```python
from build123d import *

# Parameters (mm, degrees)
SKETCH1_W                       = 101.6
SKETCH1_H                       = 114.3
BOSS_EXTRUDE1_DEPTH             = 19.05
SKETCH2_R                       = 30.999938
CUT_EXTRUDE1_DEPTH              = 7.62
SKETCH4_R                       = 15.875
CUT_EXTRUDE2_DEPTH              = 155.110195964
SKETCH5_R                       = 4.0005
CUT_EXTRUDE4_DEPTH              = 155.110195964
SKETCH10_R                      = 7.12499972
CUT_EXTRUDE5_DEPTH              = 7.62
TAP_DRILL_FOR_M8X1_0_TAP2_D     = 7
TAP_DRILL_FOR_M8X1_0_TAP2_DEPTH = 25.4
TAP_DRILL_FOR_M8X1_0_TAP2_TIP   = 2.103012167
TAP_DRILL_FOR_M8X1_0_TAP3_D     = 7
TAP_DRILL_FOR_M8X1_0_TAP3_DEPTH = 25.4
TAP_DRILL_FOR_M8X1_0_TAP3_TIP   = 2.103012167


with BuildPart() as part:
    # Sketch1 → Boss-Extrude1 (new body)
    with BuildSketch(Plane.YZ):
        with Locations((50.8, 57.15)):
            Rectangle(SKETCH1_W, SKETCH1_H)
    extrude(amount=BOSS_EXTRUDE1_DEPTH)

    # Sketch2 → Cut-Extrude1 (cut)
    with BuildSketch(Plane.YZ.offset(19.05)):
        with Locations(Location((50.8, 57.15, 0), (0, 0, 270))):
            Circle(SKETCH2_R)
    extrude(amount=-CUT_EXTRUDE1_DEPTH, mode=Mode.SUBTRACT)

    # Sketch4 → Cut-Extrude2 (cut, through all)
    with BuildSketch(Plane(origin=(0, 0, 0), x_dir=(0, -1, 0), z_dir=(-1, 0, 0))):
        with Locations(Location((-50.8, 57.15, 0), (0, 0, 90))):
            Circle(SKETCH4_R)
    extrude(amount=-CUT_EXTRUDE2_DEPTH, mode=Mode.SUBTRACT)

    # Sketch5 → Cut-Extrude4 (cut, through all)
    with BuildSketch(Plane.YZ.offset(19.05)):
        with Locations(Location((8.382, 99.568, 0), (0, 0, 270))):
            Circle(SKETCH5_R)
        with Locations(Location((93.218, 99.568, 0), (0, 0, 270))):
            Circle(SKETCH5_R)
        with Locations(Location((93.218, 14.732, 0), (0, 0, 270))):
            Circle(SKETCH5_R)
        with Locations(Location((8.382, 14.732, 0), (0, 0, 270))):
            Circle(SKETCH5_R)
    extrude(amount=-CUT_EXTRUDE4_DEPTH, mode=Mode.SUBTRACT)

    # Sketch10 → Cut-Extrude5 (cut)
    with BuildSketch(Plane.YZ.offset(19.05)):
        with Locations(Location((8.382, 99.568, 0), (0, 0, 270))):
            Circle(SKETCH10_R)
        with Locations(Location((93.218, 99.568, 0), (0, 0, 270))):
            Circle(SKETCH10_R)
        with Locations(Location((93.218, 14.732, 0), (0, 0, 270))):
            Circle(SKETCH10_R)
        with Locations(Location((8.382, 14.732, 0), (0, 0, 270))):
            Circle(SKETCH10_R)
    extrude(amount=-CUT_EXTRUDE5_DEPTH, mode=Mode.SUBTRACT)

    # Tap Drill for M8x1.0 Tap2
    with Locations(Plane.XY.offset(114.3)):
        with Locations((9.398, 73.152), (9.398, 28.448)):
            Hole(TAP_DRILL_FOR_M8X1_0_TAP2_D / 2, depth=TAP_DRILL_FOR_M8X1_0_TAP2_DEPTH)
            with Locations((0, 0, -(TAP_DRILL_FOR_M8X1_0_TAP2_DEPTH + TAP_DRILL_FOR_M8X1_0_TAP2_TIP / 2))):  # 118° drill point
                Cone(0, TAP_DRILL_FOR_M8X1_0_TAP2_D / 2, TAP_DRILL_FOR_M8X1_0_TAP2_TIP, mode=Mode.SUBTRACT)

    # Tap Drill for M8x1.0 Tap3
    with Locations(Plane(origin=(0, 0, 0), x_dir=(1, 0, 0), z_dir=(0, 0, -1))):
        with Locations((9.398, -73.152), (9.398, -28.448)):
            Hole(TAP_DRILL_FOR_M8X1_0_TAP3_D / 2, depth=TAP_DRILL_FOR_M8X1_0_TAP3_DEPTH)
            with Locations((0, 0, -(TAP_DRILL_FOR_M8X1_0_TAP3_DEPTH + TAP_DRILL_FOR_M8X1_0_TAP3_TIP / 2))):  # 118° drill point
                Cone(0, TAP_DRILL_FOR_M8X1_0_TAP3_D / 2, TAP_DRILL_FOR_M8X1_0_TAP3_TIP, mode=Mode.SUBTRACT)


solid = part.part
```
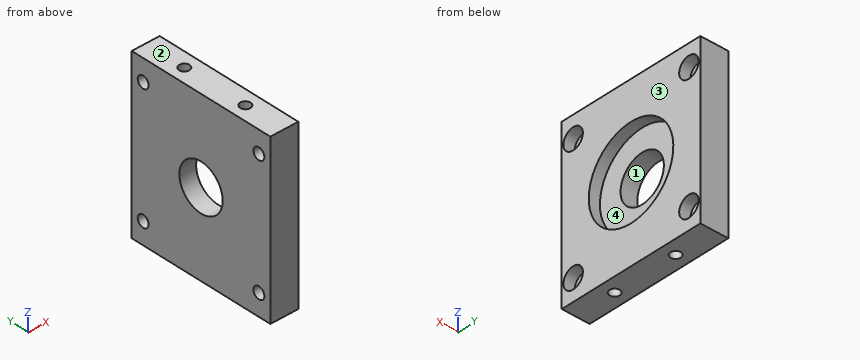
Here's how the part is built. I have some questions about the finished solid (model axes, mm). Face numbers are marked on the shaded views. Give positions to 0.01 mm unless a question says otherwise; leave off trailing zeros. Write each loop counter-clockwise with the first axis right and the second up, starting at its lowest first coordinate (ties: lowest second). Pieces come first, ordered by that corner, then holes.
(1) If I drill on L1, parallel to Y at x = 17, z = 57.15; L2, parallel to Y at x = 5, z = 70; L3, parallel to X at y = 65.5, z = 66.5, over which ranges is the centre line in solid material (lowest first)?
Output values:
L1: y = 0 to 19.8, 81.8 to 101.6
L2: y = 0 to 41.48, 60.12 to 101.6
L3: x = 0 to 11.43
(2) Thinking about a two-plate mould opening in Z: for the marked faces 1, 2, 3 and 4, which applies, pulls with the +Z half, pulls with the -Z half, needs draft (parallel to the pull), parting line crosses it, or undercut?
Output values:
face 1: undercut
face 2: pulls with the +Z half
face 3: needs draft
face 4: undercut
(3) Will these pins go through, and if not, where does the flat tip stop? pin 1 (4 mm diameter, centred on y = 22.5, z = 60.5, fed in from +X); pin 2 (5.5 mm diameter, centred on x = 9.398, y = 28.448, fed in from -Z).
Output values:
pin 1: stops at x = 11.43
pin 2: stops at z = 25.85
(4) Imagine slicing it at C-C, the plane z = 14. Write out the boundary of the cut face in (x, y).
Output values:
outline: (0, 0) - (19.05, 0) - (19.05, 1.29) - (11.43, 1.29) - (11.43, 4.45) - (0, 4.45) - close; (0, 12.31) - (11.43, 12.31) - (11.43, 15.47) - (19.05, 15.47) - (19.05, 86.13) - (11.43, 86.13) - (11.43, 89.29) - (0, 89.29) - close; (0, 97.15) - (11.43, 97.15) - (11.43, 100.31) - (19.05, 100.31) - (19.05, 101.6) - (0, 101.6) - close; hole circle Ø7 at (9.4, 28.45); hole circle Ø7 at (9.4, 73.15)
(5) Imagine slicing it at D-D, the plane x = 16.5. Write out the boundary of the cut face in (y, z) (3 decimals).
Output values:
outline: (0, 0) - (101.6, 0) - (101.6, 114.3) - (0, 114.3) - close; hole circle Ø14.25 at (8.382, 14.732); hole circle Ø14.25 at (8.382, 99.568); hole circle Ø62 at (50.8, 57.15); hole circle Ø14.25 at (93.218, 14.732); hole circle Ø14.25 at (93.218, 99.568)
(6) Imagine slicing it at B-B, the plane y = 50.8. Write out the boundary of the cut face in (x, z) (3 decimals), and give its area (3 significant figures).
Output values:
outline: (0, 0) - (19.05, 0) - (19.05, 26.15) - (11.43, 26.15) - (11.43, 41.275) - (0, 41.275) - close; (0, 73.025) - (11.43, 73.025) - (11.43, 88.15) - (19.05, 88.15) - (19.05, 114.3) - (0, 114.3) - close
area: 1,340 mm2
(7) Imagine slicing it at A-A, the plane z = 57.15. Write out the boundary of the cut face in (x, y) (3 decimals), and give its area (3 significant figures).
Output values:
outline: (0, 0) - (19.05, 0) - (19.05, 19.8) - (11.43, 19.8) - (11.43, 34.925) - (0, 34.925) - close; (0, 66.675) - (11.43, 66.675) - (11.43, 81.8) - (19.05, 81.8) - (19.05, 101.6) - (0, 101.6) - close
area: 1,100 mm2
